Source: three-view drawing plus pictorial views. Frame: mm from the lowest corner of the part. Coordinates: 2 decimals unless noted, no trailing zeros. Order: outer loops, then holes, each group sorted by start corner. A loop starts at its lowest first (then second) coordinate and runs counter-clockwise, first axis right, second up. Notation, with made-up numbers: (-12, 50) - (-5, 50) arc R17 ccw to (-5, 61) - close; hole circle Ø5 at (-30.5, 20). An arc over 180 degrees is marked (long way). One line per question, with ' | ' between items.
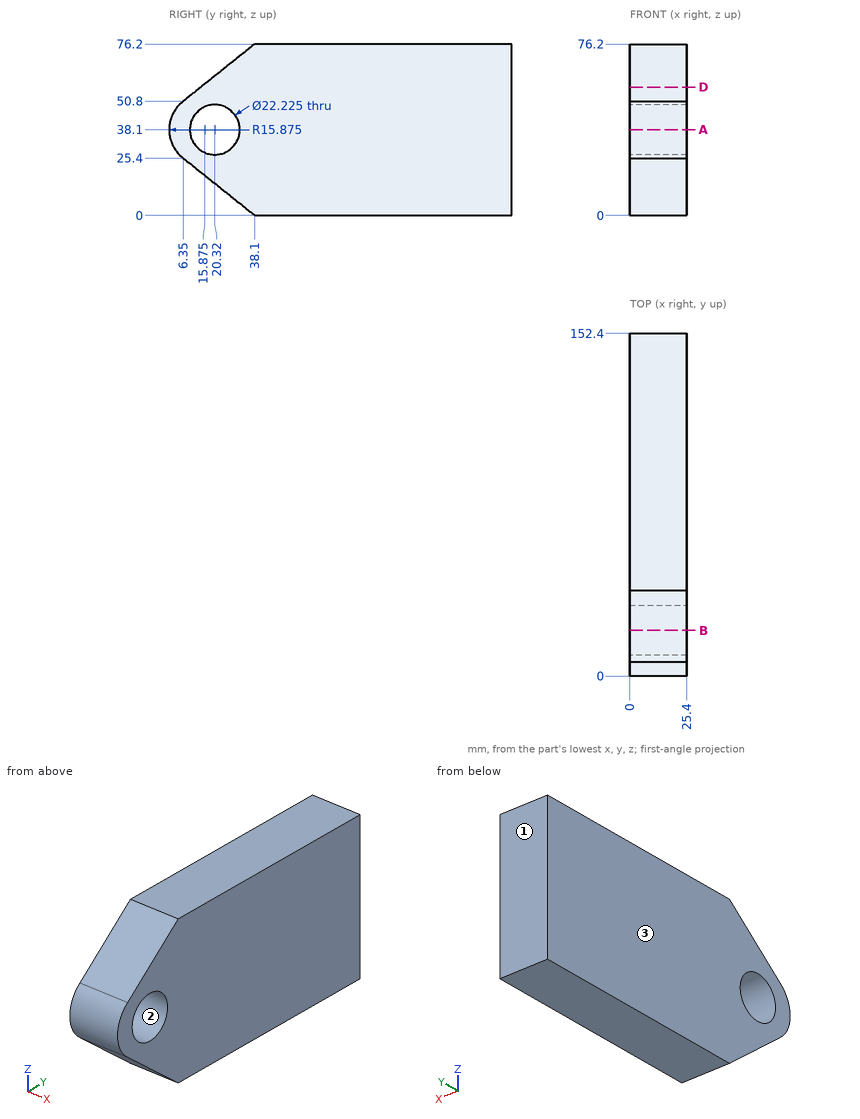
Item 1: Section D-D on z = 57. Return the cut outline in (x, y).
Data:
outline: (0, 14.1) - (25.4, 14.1) - (25.4, 152.4) - (0, 152.4) - close
Item 2: Contact query for flat-ended pins moving along their axis: P1, Ø8, axis at x = 4, y = 72, coming from the -Z side; P2, Ø3, axis at x = 7, z = 32, coming from the -Y side. Output: stop coordinate, or through.
Data:
P1: z = 0 | P2: y = 0.68
Item 3: Section A-A on z = 38.1. Return the cut outline in (x, y).
Data:
outline: (0, 0) - (25.4, 0) - (25.4, 9.21) - (0, 9.21) - close; (0, 31.43) - (25.4, 31.43) - (25.4, 152.4) - (0, 152.4) - close
Item 4: Ray query, line 1 (Y direction, x = 1, z = 37.5); line 2 (Y direction, x = 8.5, z = 41); line 3 (Z direction, x = 18, y = 20.32). Return the intervals inside material, ascending.
Data:
line 1: 0.01 to 9.22, 31.42 to 152.4 | line 2: 0.27 to 9.59, 31.05 to 152.4 | line 3: 14.22 to 26.99, 49.21 to 61.98
Item 5: Section B-B on y = 20.32. Return the cut outline in (x, z), and give its area (3 significant figures).
Data:
outline: (0, 14.22) - (25.4, 14.22) - (25.4, 26.99) - (0, 26.99) - close; (0, 49.21) - (25.4, 49.21) - (25.4, 61.98) - (0, 61.98) - close | area: 648 mm^2
Item 6: Draft query along Y for the marked faces 1, 2 and 3. Return one class per face: released by +Y, released by -Y, zero draft, split by the parting line, or undercut.
Data:
face 1: released by +Y | face 2: undercut | face 3: zero draft
